Source: CAD feature listing. Evaluate the final solid. Frame: model axes, mm. A direction names the side the tool comes from. Coordinates: 2 decimals unless noted, no trailing zeros. Write each loop counter-clockwise with the first axis right and the second up, starting at its lowest first coordinate (ties: lowest second). Pieces come first, ordered by that corner, then holes. Notation, with made-up numbers: (-23.75, 53.25) - (-9.75, 53.25) arc R15 ccw to (-9.75, 58.25) - close; hole circle Ø10 at (38, 19.5). An arc over 180 degrees is marked (long way). One line per item, written item: value.
from build123d import *

# Parameters (mm, degrees)
SKETCH_1_R               = 21
SKETCH_1_R_2             = 1.5
EXTRUDE_1_DEPTH          = 10
SKETCH_2_R               = 14
EXTRUDE_2_DEPTH          = 3.5
SKETCH_3_R               = 10
EXTRUDE_3_DEPTH          = 8.5
SKETCH_5_R               = 2
CUT_EXTRUDE_1_DEPTH      = 28
SKETCH_4_R               = 1.4
CUT_EXTRUDE_2_DEPTH      = 9.5
CUT_EXTRUDE_3_DEPTH      = 15.5
CUT_EXTRUDE_3_DEPTH_BACK = 5.5
SKETCH_6_R               = 4


with BuildPart() as part:
    # 草图1 → 凸台-拉伸1 (new body)
    with BuildSketch(Plane.XY):
        Circle(SKETCH_1_R)
        with Locations((0, -15.5)):
            Circle(SKETCH_1_R_2, mode=Mode.SUBTRACT)
        with Locations((-15.5, 0)):
            Circle(SKETCH_1_R_2, mode=Mode.SUBTRACT)
        with Locations((0, 15.5)):
            Circle(SKETCH_1_R_2, mode=Mode.SUBTRACT)
        with Locations((15.5, 0)):
            Circle(SKETCH_1_R_2, mode=Mode.SUBTRACT)
    extrude(amount=EXTRUDE_1_DEPTH)

    # 草图2 → 凸台-拉伸2 (add)
    with BuildSketch(Plane(origin=(0, 0, 0), x_dir=(-1, 0, 0), z_dir=(0, 0, -1))):
        with Locations((0, -3.5)):
            Circle(SKETCH_2_R)
    extrude(amount=EXTRUDE_2_DEPTH)

    # 草图3 → 凸台-拉伸3 (add)
    with BuildSketch(Plane(origin=(0, 0, -3.5), x_dir=(-1, 0, 0), z_dir=(0, 0, -1))):
        with Locations((0, -3.5)):
            Circle(SKETCH_3_R)
    extrude(amount=EXTRUDE_3_DEPTH)

    # 草图5 → 切除-拉伸1 (cut)
    with BuildSketch(Plane.XY.offset(10)):
        Circle(SKETCH_5_R)
    extrude(amount=-CUT_EXTRUDE_1_DEPTH, mode=Mode.SUBTRACT)

    # 草图4 → 切除-拉伸2 (cut)
    with BuildSketch(Plane(origin=(0, 0, -12), x_dir=(-1, 0, 0), z_dir=(0, 0, -1))):
        with Locations((-6.5, 0)):
            Circle(SKETCH_4_R)
        with Locations(Location((6.5, 0, 0), (0, 0, 180))):
            Circle(SKETCH_4_R)
    extrude(amount=-CUT_EXTRUDE_2_DEPTH, mode=Mode.SUBTRACT)

    # 草图6 → 切除-拉伸3 (cut, two sides: drawn at the far end of the back side and taken through both)
    with BuildSketch(Plane(origin=(0, 0, 0), x_dir=(-1, 0, 0), z_dir=(0, 0, -1)).offset(-CUT_EXTRUDE_3_DEPTH_BACK)):
        with Locations(Location((0, 15.5, 0), (0, 0, 180))):
            Circle(SKETCH_6_R)
        with Locations(Location((15.5, 0, 0), (0, 0, 137.496782389))):
            Circle(SKETCH_6_R)
        with Locations(Location((0, -15.5, 0), (0, 0, 202.024312837))):
            Circle(SKETCH_6_R)
        with Locations(Location((-15.5, 0, 0), (0, 0, 292.048071018))):
            Circle(SKETCH_6_R)
    extrude(amount=CUT_EXTRUDE_3_DEPTH + CUT_EXTRUDE_3_DEPTH_BACK, mode=Mode.SUBTRACT)


solid = part.part
1) Contact query for flat-ended pins moving along their axis: P1, Ø2.5, axis at x = 1.5, y = -17, coming from the -Z side; P2, Ø9, axis at x = -1.5, y = 14.5, coming from the -Z side; P3, Ø1.5, axis at y = -7.5, z = -9, coming from the +X side; P4, Ø1.8, axis at x = 15.5, y = 0, coming from the +Z side. Output: stop coordinate, or through.
Values found:
P1: z = 5.5
P2: z = -3.5
P3: x = 9.46
P4: through
2) Section query A-A on x = 0. Output: boundary loops of the cut face in (y, z), then the cut area to 3 significant figures.
Values found:
outline: (-21, 0) - (-19.5, 0) - (-19.5, 5.5) - (-17, 5.5) - (-17, 10) - (-21, 10) - close; (-14, 5.5) - (-11.5, 5.5) - (-11.5, -12) - (-2, -12) - (-2, 10) - (-14, 10) - close; (2, -12) - (6.5, -12) - (6.5, -3.5) - (10.5, -3.5) - (10.5, 0) - (11.5, 0) - (11.5, 5.5) - (14, 5.5) - (14, 10) - (2, 10) - close; (17, 5.5) - (19.5, 5.5) - (19.5, 0) - (21, 0) - (21, 10) - (17, 10) - close
area: 447 mm2
3) Reachability of faces 1 (the cylindrical face through (-7.9, -0.06, -7.32)), 2 (the cylindrical face through (-17, 0, 8)), 3 (the cylindrical face through (-0.2, 10.5, -1.7)) from +Z, -Z, +X, -X, +Y, -Y: full face, straight path, thin tool, end or side. Return the list, or none.
Values found:
face 1: -Z
face 2: +Z, -Z
face 3: -Z, +Y
4) Section query B-B on y = 15.5. Output: boundary loops of the cut face in (x, z), then the cut area to 3 significant figures.
Values found:
outline: (-14.17, 0) - (-4, 0) - (-4, 5.5) - (-1.5, 5.5) - (-1.5, 10) - (-14.17, 10) - close; (1.5, 5.5) - (4, 5.5) - (4, 0) - (14.17, 0) - (14.17, 10) - (1.5, 10) - close
area: 226 mm2
5) Draft query along X for faces 4 (the cylindrical face through (14, 0, 8)), 5 (the cylindrical face through (-11.636, -1.034, 2.063)), 6 (the flat face through (4, 6, -3.5)), 7 (the cylindrical face through (20.03, 6.31, 4.93)). Return one class per face: released by +X, released by -X, zero draft, split by the parting line, or undercut.
Values found:
face 4: undercut
face 5: undercut
face 6: zero draft
face 7: split by the parting line
6) Material intervals for line 1 (X direction, y = -2.5, z = 1); line 2 (Z direction, x = 1, y = 18); line 3 (Z direction, x = -11, y = -11.5), sorted ascending.
Values found:
line 1: -20.85 to -18.62, -12.38 to 12.38, 18.62 to 20.85
line 2: 5.5 to 10
line 3: -3.5 to 10
7) Section query C-C on z = 3.75. Output: boundary loops of the cut face in (x, y).
Values found:
outline: circle Ø42 at (0, 0); hole circle Ø8 at (-15.5, 0); hole circle Ø8 at (0, -15.5); hole circle Ø8 at (0, 15.5); hole circle Ø4 at (0, 0); hole circle Ø8 at (15.5, 0)
